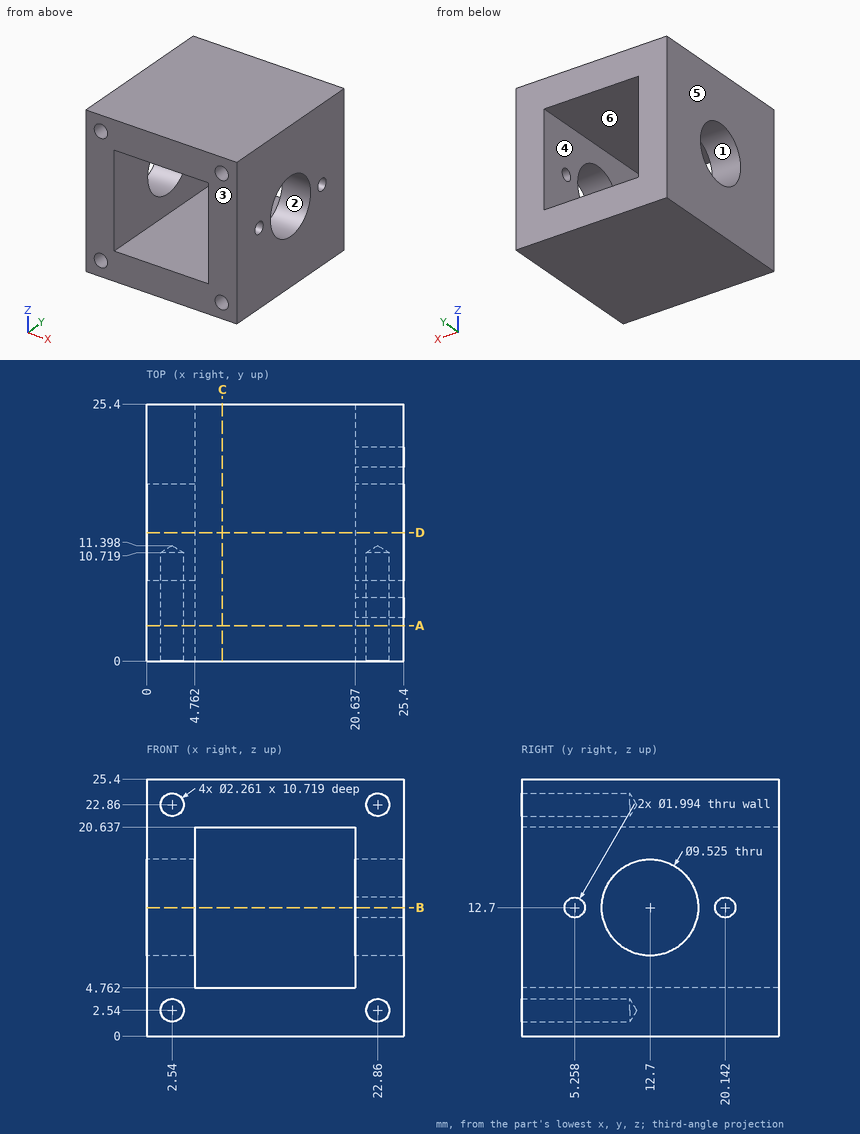
Drawing for the job (mm, zero at the part's lowest x, y, z). A direction names the side the tool comes from. Give positions to 0.01 mm unless a question says otherwise; leave off trailing zeros. Loops run counter-clockwise (first coordinate to the right, second up) from the corner with the lowest first, then second, coordinate; pieces in that order, holes last.
(1) Pull direction Y, two halves, no side cores. Call the marked faces 1, 2, 3 and 4: pulls with the +Y half, pulls with the -Y half, needs draft (parallel to the pull), parting line crosses it, or undercut.
Return value:
face 1: undercut
face 2: undercut
face 3: pulls with the -Y half
face 4: needs draft
(2) Band-saw the part on D-D (y = 12.7). Write the cut outline in (x, z).
Return value:
outline: (0, 0) - (25.4, 0) - (25.4, 7.94) - (20.64, 7.94) - (20.64, 4.76) - (4.76, 4.76) - (4.76, 7.94) - (0, 7.94) - close; (0, 17.46) - (4.76, 17.46) - (4.76, 20.64) - (20.64, 20.64) - (20.64, 17.46) - (25.4, 17.46) - (25.4, 25.4) - (0, 25.4) - close
(3) Band-saw the part on A-A (y = 3.5). Write the cut outline in (x, z).
Return value:
outline: (0, 0) - (25.4, 0) - (25.4, 25.4) - (0, 25.4) - close; hole circle Ø2.26 at (2.54, 2.54); hole circle Ø2.26 at (2.54, 22.86); hole (4.76, 4.76) - (20.64, 4.76) - (20.64, 20.64) - (4.76, 20.64) - close; hole circle Ø2.26 at (22.86, 2.54); hole circle Ø2.26 at (22.86, 22.86)
(4) Band-saw the part on C-C (x = 7.5). Write the cut outline in (y, z), and give its area (3 significant figures).
Return value:
outline: (0, 0) - (25.4, 0) - (25.4, 4.76) - (0, 4.76) - close; (0, 20.64) - (25.4, 20.64) - (25.4, 25.4) - (0, 25.4) - close
area: 242 mm2
(5) Band-saw the part on B-B (z = 12.7). Write the cut outline in (x, y) (1 decimal), and give its area (3 significant figures).
Return value:
outline: (0, 0) - (4.8, 0) - (4.8, 7.9) - (0, 7.9) - close; (0, 17.5) - (4.8, 17.5) - (4.8, 25.4) - (0, 25.4) - close; (20.6, 0) - (25.4, 0) - (25.4, 4.3) - (20.6, 4.3) - close; (20.6, 6.3) - (25.4, 6.3) - (25.4, 7.9) - (20.6, 7.9) - close; (20.6, 17.5) - (25.4, 17.5) - (25.4, 19.1) - (20.6, 19.1) - close; (20.6, 21.1) - (25.4, 21.1) - (25.4, 25.4) - (20.6, 25.4) - close
area: 132 mm2
(6) Drill centre lines: line 1 along Y through (x, z) = (21.85, 12.7) (1 decimal); line 2 along Z through (x, y) = (22.86, 2.5). Where is each one in solid material? Low to high.
Return value:
line 1: y = 0 to 4.3, 6.3 to 7.9, 17.5 to 19.1, 21.1 to 25.4
line 2: z = 0 to 1.41, 3.67 to 21.73, 23.99 to 25.4
(7) 3-axis set-ups, long thin cutter, end or side, ignore diameter. For the marked faces 5 and 6: which of +Z, -Z, +X, -X, +Y, -Y reach the whole face in a straight line?
Return value:
face 5: +Z, -Z, -X, +Y, -Y
face 6: +Y, -Y
(8) Pin check, flat tip, straight feed: pin 1 (7.5 mm diameter, centred on y = 12.7, z = 12.7, fed in from +X). Stop position of the tip, or through.
Return value:
pin 1: passes through
